Autodesk Inventor part; units mm, degrees
ref_plane "YZ Plane" through (0, 0, 0) normal (1, 0, 0) x (0, 1, 0)
ref_plane "XZ Plane" through (0, 0, 0) normal (0, 1, 0) x (-1, 0, 0)
ref_plane "XY Plane" through (0, 0, 0) normal (0, 0, 1) x (1, 0, 0)
sketch "Sketch1" plane through (0, 0, 0) normal (0, 1, 0) x (-1, 0, 0)
  line L0 (0, 0) -> (10, 0)
  line L1 (10, 0) -> (10, -25)
  line L2 (10, -25) -> (0, -25)
  line L3 (0, -25) -> (0, 0)
  dimension "d0" = 10
  dimension "d1" = 25
extrude "Extrusion1" add sketch "Sketch1" along normal blind 2
sketch "Sketch2" plane through (0, 2, 0) normal (0, 1, 0) x (1, 0, 0)
  line L0 (-10, 0) -> (0, 0)
  line L1 (-10, 0) -> (-10, 1)
  line L2 (-10, 1) -> (-7, 1)
  line L3 (-7, 1) -> (-7, 4)
  line L4 (-7, 4) -> (-10, 4)
  line L5 (-10, 4) -> (-10, 1)
  line L6 (0, 25) -> (-10, 25)
  line L7 (-10, 25) -> (-10, 24)
  line L8 (-10, 24) -> (-7, 24)
  line L9 (-7, 24) -> (-7, 21)
  line L10 (-7, 21) -> (-10, 21)
  line L11 (-10, 21) -> (-10, 24)
  dimension "d4" = 1
  dimension "d5" = 3
  dimension "d6" = 3
  dimension "d7" = 1
  dimension "d8" = 3
  dimension "d9" = 3
extrude "Extrusion2" add sketch "Sketch2" along normal blind 10
sketch "Sketch3" plane through (-7, 2, -1) normal (1, 0, 0) x (0, 0, -1)
  line L0 (0, 0) -> (0, 10)
  line L1 (0, 10) -> (1.5, 10)
  line L2 (1.5, 10) -> (1.5, 8.5)
  line L3 (1.5, 8.5) -> (0, 8.5)
  line L4 (0, 8.5) -> (0, 10)
  line L5 (23, 10) -> (20, 10)
  line L6 (23, 10) -> (21.5, 10)
  line L7 (21.5, 10) -> (21.5, 8.5)
  line L8 (21.5, 8.5) -> (23, 8.5)
  line L9 (23, 8.5) -> (23, 10)
  circle A0 centre (1.5, 8.5) radius 1.5
  circle A1 centre (21.5, 8.5) radius 1.5
  point P0 (-1, -2)
  dimension "d12" = 1.5
  dimension "d13" = 1.5
  dimension "d14" = 1.5
  dimension "d15" = 1.5
  dimension "d16" = 3
  dimension "d17" = 3
extrude "Extrusion3" add sketch "Sketch3" along normal blind 3 contours A0 L2 L3 | L3 L2 A0 | A1 L8 L7 | L7 L8 A1
sketch "Sketch4" plane through (0, 2, 0) normal (0, 1, 0) x (1, 0, 0)
  line L0 (0, 0) -> (-5, 0)
  line L1 (-5, 0) -> (-5, 12.5)
  line L2 (-5, 12.5) -> (0, 12.5)
  line L3 (0, 12.5) -> (0, 0)
  circle A0 centre (-5, 12.5) radius 1.125
  dimension "d20" = 5
  dimension "d21" = 12.5
  dimension "d22" = 2.25
extrude "Extrusion4" cut sketch "Sketch4" against normal blind 2 contours A0 L2 L1 | L1 L2 A0
properties part number "LaserMountTop"
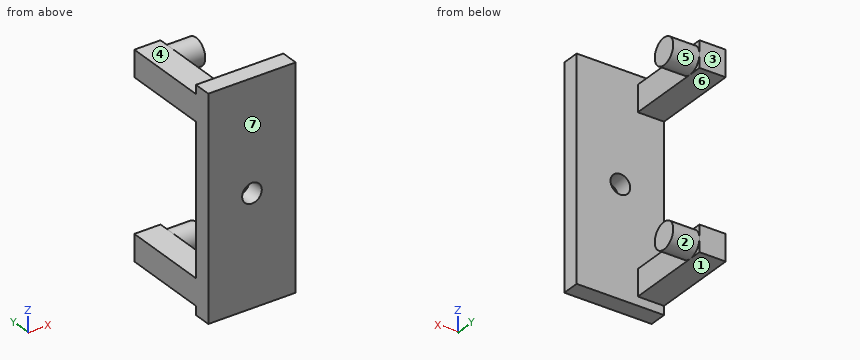
The model under review builds one solid part; all positions refer to its coordinate system, in mm. Face numbers are marked on the shaded views. A direction names the side the tool comes from. Give positions to 0.01 mm unless a question says otherwise; leave off trailing zeros. Write each loop counter-clockwise with the first axis right and the second up, starting at its lowest first coordinate (ties: lowest second). Pieces come first, ordered by that corner, then holes. Notation, with made-up numbers: M 54.25,71.5 L 76.25,71.5 A22 ccw 76.25,83.5 Z; hole C 89.5,21 d9. An arc over 180 degrees is marked long. Write item = value, one per line. Start each with the question number.
Q1. Mouldability with a two-part tool opening along Z and no side actions: class the marked faces 1, 2 and 3 as released by +Z, released by -Z, zero draft, split by the parting line, or undercut.
Q2. For line 1 (Z direction, x = -5, y = 1.4) (3 decimals); line 2 (Z direction, x = -9, y = 10); line 3 (X direction, y = 0.9, z = -12.5) (3 decimals), list the stretches that pass through material, from the lowest coordinate up.
Q3. We need section D-D (z = -15.5). State the section outline as (x, y) points.
Q4. Machinability: for the marked faces 4, 5, 6 and 7, which of the approach directions +Z, -Z, +X, -X, +Y, -Y give a long, thin tool a straight path to every point of the face, cutting with its end or side? Answer none if there is none.
Q5. We need section C-C (z = -13). State the section outline as (x, y) points, plus the area to 3 significant figures.
Q6. We need section B-B (x = -5). State the section outline as (y, z) points (3 decimals), plus the area to 3 significant figures.
Q7. Clearance check with flat-ended pins moving along their axes: pin 1 (0.8 mm diameter, centred on y = 11, z = -23, fed in from +X); pin 2 (2.5 mm diameter, centred on x = -9, y = 6.5, fed in from -Z); pin 3 (1 mm diameter, centred on x = -1.5, y = 3, fed in from +Z); pin 4 (1.5 mm diameter, centred on y = 6.5, z = -23, fed in from +X). State where each tip first meets the part, or that it passes through.
Q8. We need section A-A (y = 2.25). State the section outline as (x, z) points.
Result set:
q1.face_1 = released by -Z
q1.face_2 = undercut
q1.face_3 = zero draft
q2.line_1 = -25 to -13.625, -11.375 to 0
q2.line_2 = -24 to -21, -4 to -1
q2.line_3 = -10 to -6.125, -3.875 to 0
q3.outline = M -10,0 L 0,0 L 0,2 L -10,2 Z
q4.face_4 = +Z, +X, -X, +Y
q4.face_5 = +X
q4.face_6 = +X, -X, +Y
q4.face_7 = +Z, -Z, +X, -X, -Y
q5.outline = M -10,0 L -6.01,0 L -6.01,2 L -10,2 Z; M -3.99,0 L 0,0 L 0,2 L -3.99,2 Z
q5.area = 16.0 mm2
q6.outline = M 0,-25 L 2,-25 L 2,-13.625 L 0,-13.625 Z; M 0,-11.375 L 2,-11.375 L 2,0 L 0,0 Z; C 10.5,-22.5 d3; C 10.5,-2.5 d3
q6.area = 59.6 mm2
q7.pin_1 = -4
q7.pin_2 = -24
q7.pin_3 = through
q7.pin_4 = -7
q8.outline = M -10,-24 L -7,-24 L -7,-21 L -10,-21 Z; M -10,-4 L -7,-4 L -7,-1 L -10,-1 Z
